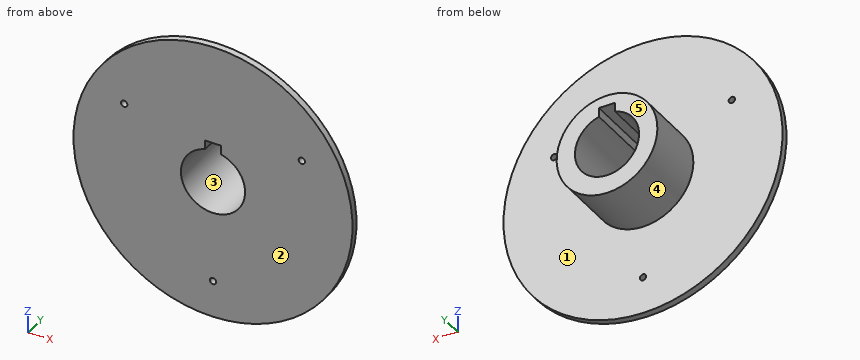
from build123d import *

# Parameters (mm, degrees)
F_1_8_0_125_DIAMETER_HOLE1_D = 3.175
CIRPATTERN2_COUNT            = 3
CIRPATTERN1_COUNT            = 3
CUT_EXTRUDE2_DEPTH           = 105.059003061


with BuildPart() as part:
    # Sketch1 → Revolve1 (revolve)
    with BuildSketch(Plane.XY, mode=Mode.PRIVATE) as revolve1_sk:
        Polygon((69.512129733, 0), (16, 0), (16, 34.123360884), (25.099562902, 34.123360884), (25.099562902, 3.412336088), (69.512129733, 3.412336088), align=None)
    revolve(revolve1_sk.sketch.rotate(Axis((0, 0, 0), (0, 1, 0)), 90), axis=Axis((0, 0, 0), (0, 1, 0)))

    # 1/8 (0.125) Diameter Hole1 (through all)
    with Locations(Plane(origin=(0, 3.412336088, -51.1125), x_dir=(0, 0, 1), z_dir=(0, 1, 0))):
        with Locations((0, 0)):
            f_1_8_0_125_diameter_hole1 = Hole(F_1_8_0_125_DIAMETER_HOLE1_D / 2)

    # CirPattern2: 1/8 (0.125) Diameter Hole1 ×3 about axis
    cirpattern2_axis = Axis((0, 0, 0), (0, 1, 0))
    for i in range(1, CIRPATTERN2_COUNT):
        add(f_1_8_0_125_diameter_hole1.rotate(cirpattern2_axis, i * 360 / CIRPATTERN2_COUNT), mode=Mode.SUBTRACT)

    # CirPattern1: 1/8 (0.125) Diameter Hole1 ×3 about axis
    cirpattern1_axis = Axis((0, 3.412336088, 0), (0, -1, 0))
    for i in range(1, CIRPATTERN1_COUNT):
        add(f_1_8_0_125_diameter_hole1.rotate(cirpattern1_axis, i * 360 / CIRPATTERN1_COUNT), mode=Mode.SUBTRACT)

    # Sketch4 → Cut-Extrude2 (cut, through all)
    with BuildSketch(Plane(origin=(0, 34.123360884, 0), x_dir=(1, 0, 0), z_dir=(0, 1, 0))):
        Polygon((0, -20), (4, -20), (4, -14.234250842), (-4, -14.234250842), (-4, -20), align=None)
    extrude(amount=-CUT_EXTRUDE2_DEPTH, mode=Mode.SUBTRACT)


solid = part.part
Geometry check sheet. Reference: the model listing, model coordinates, mm. Face numbers are marked on the shaded views. A direction names the side the tool comes from. Give positions to 0.01 mm unless a question says otherwise; leave off trailing zeros. Order: outer loops, then holes, each group sorted by start corner. A loop starts at its lowest first (then second) coordinate and runs counter-clockwise, first axis right, second up.
1) Tool access check on the marked faces 1 and 2. Record the directions out of +Z, -Z, +X, -X, +Y, -Y that give a thin tool (end or side, any length) a straight path to the whole face; none if there is none.
Results are:
face 1: +Y
face 2: +Z, -Z, +X, -X, -Y
2) Material ranges on probe 1 along X at (y, z) = (22, 0); probe 2 along Y at (x, z) = (-58, -19.5); probe 3 along X at (y, z) = (17, -4), recorded low to high.
Results are:
probe 1: x = -25.1 to -16, 16 to 25.1
probe 2: y = 0 to 3.41
probe 3: x = -24.78 to -15.49, 15.49 to 24.78
3) Cross-section at A-A (z = 0). Record the boundary of the cut face in (x, y).
Results are:
outline: (-69.51, 0) - (-16, 0) - (-16, 34.12) - (-25.1, 34.12) - (-25.1, 3.41) - (-69.51, 3.41) - close; (16, 0) - (69.51, 0) - (69.51, 3.41) - (25.1, 3.41) - (25.1, 34.12) - (16, 34.12) - close
4) Gauge pin test, flat ends, axial feed: pin 1 (5 mm diameter, centred on y = 17, z = 18, fed in from +X); pin 2 (3.5 mm diameter, centred on y = 22, z = 18, fed in from -X); pin 3 (4 mm diameter, centred on x = 44.26, z = 25.56, fed in from +Y). Record the tip position at first contact, or that the pin passes through.
Results are:
pin 1: stops at x = 19.74
pin 2: stops at x = -19.13
pin 3: stops at y = 3.41
5) Cross-section at B-B (y = 22). Record the boundary of the cut face in (x, z), then the cut area to 3 significant figures.
Results are:
outline: circle Ø50.2 at (0, 0); hole (-4, 15.49) arc R16 ccw (long way) to (4, 15.49) - (4, 20) - (-4, 20) - close
area: 1,140 mm2
6) Cross-section at D-D (x = -19.5). Record the boundary of the cut face in (y, z).
Results are:
outline: (0, -66.72) - (3.41, -66.72) - (3.41, -15.8) - (34.12, -15.8) - (34.12, 15.8) - (3.41, 15.8) - (3.41, 66.72) - (0, 66.72) - close
7) Cross-section at C-C (x = 12.5). Record the boundary of the cut face in (y, z), then the cut area to 3 significant figures.
Results are:
outline: (0, -68.38) - (3.41, -68.38) - (3.41, -21.77) - (34.12, -21.77) - (34.12, -9.99) - (0, -9.99) - close; (0, 9.99) - (34.12, 9.99) - (34.12, 21.77) - (3.41, 21.77) - (3.41, 68.38) - (0, 68.38) - close
area: 1,120 mm2
8) Draft check along Z on the marked faces 3, 4 and 5. Enter one of: released by +Z, released by -Z, zero draft, split by the parting line, or undercut.
Results are:
face 3: undercut
face 4: split by the parting line
face 5: zero draft
